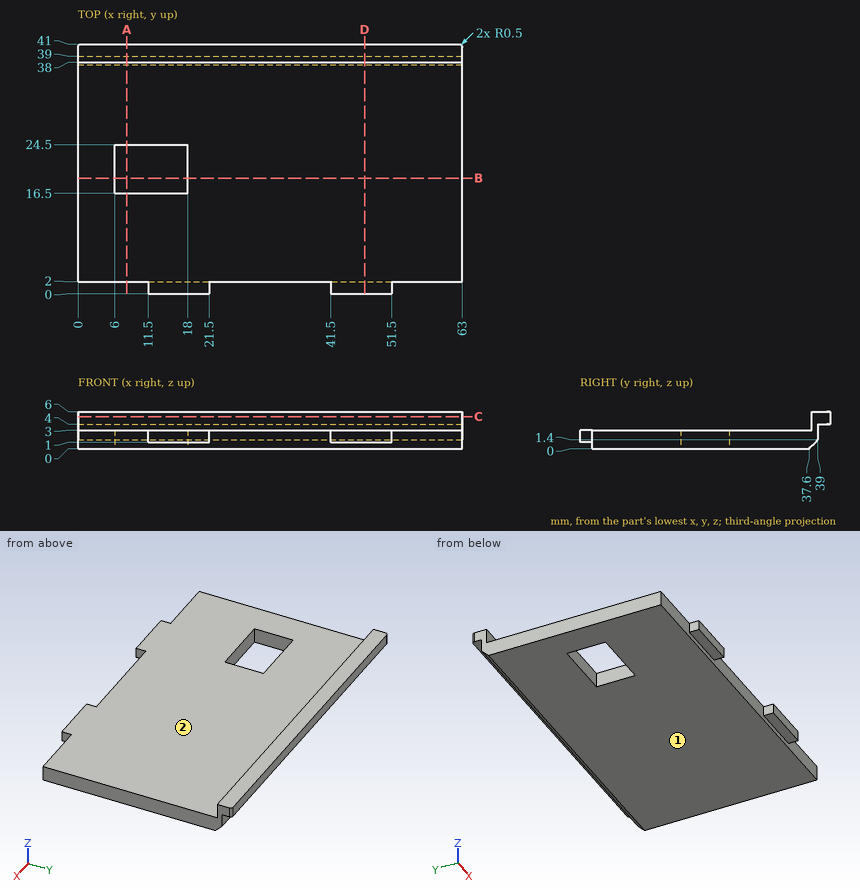
Input: dimensioned drawing with shaded views. Units: mm. Origin: part minimum x, y, z. A direction names the side the tool comes from. Coordinates: 2 decimals unless noted, no trailing zeros. Order: outer loops, then holes, each group sorted by start corner. A loop starts at its lowest first (then second) coordinate and runs counter-clockwise, first axis right, second up.
Item 1: Section query A-A (x = 8). Output: boundary loops of the cut face in (y, z).
Answer:
outline: (2, 0) - (16.5, 0) - (16.5, 3) - (2, 3) - close; (24.5, 0) - (37.6, 0) - (39, 1.4) - (39, 4) - (41, 4) - (41, 6) - (38, 6) - (38, 3) - (24.5, 3) - close
Item 2: Contact query for flat-ended pins moving along their axis: P1, Ø0.6, axis at y = 1, z = 2, coming from the -X side; P2, Ø0.6, axis at x = 46.5, y = 40, coming from the -Z side; P3, Ø2.5, axis at x = 27, z = 4.5, coming from the -Y side; P4, Ø2, axis at x = 46.5, y = 1.5, coming from the -Z side. Output: stop coordinate, or through.
Answer:
P1: stops at x = 11.5
P2: stops at z = 4
P3: stops at y = 38
P4: stops at z = 0
Item 3: Material intervals for line 1 along X through (y, z) = (20, 2); line 2 along Y through (x, z) = (35.5, 5.25); line 3 along Y through (x, z) = (25.5, 2.25), sorted ascending.
Answer:
line 1: x = 0 to 6, 18 to 63
line 2: y = 38 to 41
line 3: y = 2 to 39
Item 4: Section query C-C (z = 5.25). Output: boundary loops of the cut face in (x, y).
Answer:
outline: (0, 38) - (63, 38) - (63, 40.5) arc R0.5 ccw to (62.5, 41) - (0.5, 41) arc R0.5 ccw to (0, 40.5) - close
Item 5: Section query D-D (x = 47). Output: boundary loops of the cut face in (y, z), then the cut area to 3 significant figures.
Answer:
outline: (0, 1) - (2, 1) - (2, 0) - (37.6, 0) - (39, 1.4) - (39, 4) - (41, 4) - (41, 6) - (38, 6) - (38, 3) - (0, 3) - close
area: 121 mm2
Item 6: Section query B-B (y = 19). Output: boundary loops of the cut face in (x, z).
Answer:
outline: (0, 0) - (6, 0) - (6, 3) - (0, 3) - close; (18, 0) - (63, 0) - (63, 3) - (18, 3) - close
Item 7: Access query for the marked faces 1 and 2. Directions: +Z, -Z, +X, -X, +Y, -Y. A direction counts if a zero-diameter tool reaches every point of the face in a straight line with its end or side. Return the directions, or none.
Answer:
face 1: -Z, +X, -X, +Y, -Y
face 2: +Z, +X, -X, -Y
